from build123d import *

# Parameters (mm, degrees)
F0_W     = 15.24
F0_H     = 15.24
F1_DEPTH = 15.24
F3_D     = 2.2606
F3_DEPTH = 14.605
F3_TIP   = 0.6791527577
F6_D     = 2.2606
F6_DEPTH = 14.605
F6_TIP   = 0.6791527577
F7_D     = 2.2606
F7_DEPTH = 14.605
F7_TIP   = 0.6791527577


with BuildPart() as f1:
    # F0 (on Front) → F1 (new body)
    with BuildSketch(Plane.XZ):
        Rectangle(F0_W, F0_H)
    extrude(amount=F1_DEPTH)

    # F3
    with Locations(Plane.XZ.offset(15.24)):
        with Locations((0, 0)):
            Hole(F3_D / 2, depth=F3_DEPTH)
            with Locations((0, 0, -(F3_DEPTH + F3_TIP / 2))):  # 118° drill point
                Cone(0, F3_D / 2, F3_TIP, mode=Mode.SUBTRACT)

    # F6
    with Locations(Plane.YZ.offset(7.62)):
        with Locations((-7.62, 0)):
            Hole(F6_D / 2, depth=F6_DEPTH)
            with Locations((0, 0, -(F6_DEPTH + F6_TIP / 2))):  # 118° drill point
                Cone(0, F6_D / 2, F6_TIP, mode=Mode.SUBTRACT)

    # F7
    with Locations(Plane.XY.offset(7.62)):
        with Locations((0, -7.62)):
            Hole(F7_D / 2, depth=F7_DEPTH)
            with Locations((0, 0, -(F7_DEPTH + F7_TIP / 2))):  # 118° drill point
                Cone(0, F7_D / 2, F7_TIP, mode=Mode.SUBTRACT)


solid = f1.part
Here's how the part is built. I have some questions about the finished solid (model axes, mm). A direction names the side the tool comes from. Coordinates: 2 decimals unless noted, no trailing zeros. Write each loop counter-clockwise with the first axis right and the second up, starting at its lowest first coordinate (ties: lowest second). Pieces come first, ordered by that corner, then holes. Notation, with made-up numbers: (12.25, -17) - (53.25, -17) arc R20 ccw to (53.25, -12) - close; hole circle Ø10 at (50.5, 44.25). An arc over 180 degrees is marked (long way). Use one line per item in the form item = value.
1) Suppose I cut it at B-B, the plane x = 5.5. Write out the boundary of the cut face in (y, z).
Solved:
outline = (-15.24, -7.62) - (0, -7.62) - (0, 7.62) - (-15.24, 7.62) - close; hole circle Ø2.26 at (-7.62, 0)
2) Suppose I cut it at A-A, the plane z = 4. Write out the boundary of the cut face in (x, y).
Solved:
outline = (-7.62, -15.24) - (7.62, -15.24) - (7.62, 0) - (-7.62, 0) - close; hole circle Ø2.26 at (0, -7.62)
3) Thinking about a two-plate mould opening in Z: for faces 4 (the cylindrical face through (0.245, -11.782, -1.103)), 5 (the flat face through (2, -8, 7.62)), 6 (the cylindrical face through (-0.522, -8.623, 4.162)), which applies, released by +Z, released by -Z, zero draft, split by the parting line, or undercut?
Solved:
face_4 = undercut
face_5 = released by +Z
face_6 = zero draft
4) On a 3-axis mill with a long thin cutter (end or side, diameter ignored), from which of +Z, -Z, +X, -X, +Y, -Y can I reach the whole of each face in a straight line? I mean faces 1 (the cylindrical face through (0.245, -3.685, -1.103)), 2 (the cylindrical face through (4.162, -8.664, -0.433)), 3 (the cylindrical face through (-0.522, -8.623, -3.935)). Say none if no direction works.
Solved:
face_1 = -Y
face_2 = +X
face_3 = +Z
5) I need wall thicknesses on line 1 (X direction, y = -12.5, z = 0); line 2 (Y direction, x = -3, z = 0); line 3 (Y direction, x = 6.5, z = 0.5). Which ranges of each line are inside material? Lowest first, please.
Solved:
line_1 = -7.62 to -1.13, 1.13 to 7.62
line_2 = -15.24 to -8.75, -6.49 to 0
line_3 = -15.24 to -8.63, -6.61 to 0
